Design review of the part built by this model. Coordinates are the model's own, in mm. A direction names the side the tool comes from. Give positions to 0.01 mm unless a question says otherwise; leave off trailing zeros. Write each loop counter-clockwise with the first axis right and the second up, starting at its lowest first coordinate (ties: lowest second). Pieces come first, ordered by that corner, then holes. Notation, with made-up numbers: M -32.75,5 L -13.75,5 A19 ccw -13.75,32 Z; hole C 82,-17.75 d3. An arc over 180 degrees is marked long. Write each question's results on one line, items separated by ' | '. Start each with the question number.
from build123d import *

# Parameters (mm, degrees)
CROQUIS1_R              = 6
SALIENTE_EXTRUIR1_DEPTH = 4.75
CROQUIS1_3_R            = 13
CROQUIS1_3_R_2          = 6
SALIENTE_EXTRUIR2_DEPTH = 3
CHAFL_N1_SIZE           = 1


with BuildPart() as part:
    # Croquis1 → Saliente-Extruir1 (new body)
    with BuildSketch(Plane(origin=(0, 0, 0), x_dir=(1, 0, 0), z_dir=(0, 1, 0))):
        Circle(CROQUIS1_R)
    extrude(amount=SALIENTE_EXTRUIR1_DEPTH)

    # Croquis1_3 → Saliente-Extruir2 (add)
    with BuildSketch(Plane(origin=(0, 0, 0), x_dir=(1, 0, 0), z_dir=(0, 1, 0))):
        Circle(CROQUIS1_3_R)
        Circle(CROQUIS1_3_R_2, mode=Mode.SUBTRACT)
        Circle(CROQUIS1_3_R_2)
    extrude(amount=-SALIENTE_EXTRUIR2_DEPTH)

    # Chafl_n1
    chafl_n1_edges = [part.edges().sort_by_distance(p)[0] for p in [
        (-6, 4.75, 0),
        (-13, -3, 0),
        (-13, 0, 0),
    ]]
    chamfer(chafl_n1_edges, length=CHAFL_N1_SIZE)


solid = part.part
Q1. We need section C-C on y = 4.25. Write out the cut boundary in (x, z).
Q2. For faces 1 (the flat face through (0, 4.75, 0)), 2 (the cylindrical face through (-6, 2, 0)), list the 3-axis set-ups (+Z, -Z, +X, -X, +Y, -Y) from which the entire face can be reached by the end or side of a thin tool; tool diameter is ignored.
Q3. Wall thickness on line 1 along Y through (x, z) = (-7.5, -7.5); line 2 along Z through (x, y) = (0, -1.25); line 3 along Z through (x, y) = (-8.75, -1.5): over which ranges is each line inside the solid? List them lowest first. Write a range as from..to.
Q4. We need section D-D on y = 2.5. Write out the cut boundary in (x, z).
Q5. For pin 1 Ø3 at (y, z) = (2, -2) entering from +X; pin 2 Ø2 at (x, z) = (-4.5, 8) entering from +Y; pin 3 Ø3 at (x, y) = (5, -2) entering from -Z, all flat-tipped, find the tip position at first contact; note any pin that passes through.
Q6. We need section A-A on x = 0. Write out the cut boundary in (y, z).
Q7. We need section B-B on z = 0. Write out the cut boundary in (x, y), and give its area (3 significant figures).
Answer sheet:
1) outline: C 0,0 d11
2) face 1: +Z, -Z, +X, -X, +Y | face 2: +Y
3) line 1: -3..0 | line 2: -13..13 | line 3: -9.61..9.61
4) outline: C 0,0 d12
5) pin 1: x = 5.98 | pin 2: y = 0 | pin 3: z = -12.52
6) outline: M -3,-12 L -2,-13 L -1,-13 L 0,-12 L 0,-6 L 3.75,-6 L 4.75,-5 L 4.75,5 L 3.75,6 L 0,6 L 0,12 L -1,13 L -2,13 L -3,12 Z
7) outline: M -13,-2 L -12,-3 L 12,-3 L 13,-2 L 13,-1 L 12,0 L 6,0 L 6,3.75 L 5,4.75 L -5,4.75 L -6,3.75 L -6,0 L -12,0 L -13,-1 Z | area: 132 mm^2
